Autodesk Inventor part; units mm, degrees
ref_plane "YZ Plane" through (0, 0, 0) normal (1, 0, 0) x (0, 1, 0)
ref_plane "XZ Plane" through (0, 0, 0) normal (0, 1, 0) x (-1, 0, 0)
ref_plane "XY Plane" through (0, 0, 0) normal (0, 0, 1) x (1, 0, 0)
sketch "Skizze1" plane through (0, 0, 0) normal (0, 0, 1) x (1, 0, 0)
  line L0 (5, 5) -> (5, 50)
  line L1 (5, 50) -> (0, 50)
  line L2 (0, 50) -> (0, 0)
  line L3 (5, 5) -> (50, 5)
  line L4 (50, 5) -> (50, 0)
  line L5 (-10, 0) -> (60, 0)
  line L6 (0, -10) -> (0, 60)
  line L7 (0, 0) -> (50, 0)
  dimension "d3" = 5
  dimension "d4" = 5
  dimension "d5" = 50
  dimension "d6" = 50
extrude "Extrusion1" add sketch "Skizze1" along normal blind 25
sketch "Skizze3" plane through (0, 0, 0) normal (0, -1, 0) x (1, 0, 0)
  line L0 (0, 0) -> (0, 25)
  line L1 (50, 0) -> (0, 0)
  line L2 (50, 0) -> (50, 25)
  line L3 (50, 25) -> (40, 25)
  line L4 (40, 25) -> (40, 0)
  line L5 (40, 0) -> (50, 0)
  line L6 (50, 0) -> (50, 25)
  dimension "d9" = 40
extrude "Extrusion2" cut sketch "Skizze3" against normal through all
sketch "Skizze4" plane through (0, 0, 0) normal (0, -1, 0) x (1, 0, 0)
  line L0 (40, 0) -> (40, 25)
  line L1 (40, 25) -> (0, 25)
  line L2 (0, 0) -> (0, 25)
  line L3 (5, 0) -> (5, 25)
  line L4 (40, 25) -> (5, 25)
  line L5 (5, 25) -> (5, 20.5)
  line L6 (5, 20.5) -> (40, 20.5)
  line L7 (40, 20.5) -> (40, 25)
  line L8 (5, 0) -> (40, 0)
  line L9 (40, 0) -> (40, 4.5)
  line L10 (40, 4.5) -> (5, 4.5)
  line L11 (5, 4.5) -> (5, 0)
  line L12 (0, 12.5) -> (40, 12.5)
  dimension "d12" = 16
extrude "Extrusion3" cut sketch "Skizze4" against normal through all contours L8 L3 L10 L0 | L6 L3 L1 L0
sketch "Skizze5" plane through (0, 0, 0) normal (0, -1, 0) x (1, 0, 0)
  line L0 (40, 4.5) -> (40, 20.5)
  line L1 (0, 0) -> (0, 25)
  line L2 (0, 12.5) -> (40, 12.5)
  point P0 (11, 12.5)
  point P1 (29, 12.5)
  dimension "d15" = 18
  dimension "d16" = 11
hole "Bohrung1" at (11, 0, 12.5) at (29, 0, 12.5) direction (0, 1, 0) diameter 4.5 end through all
fillet "Rundung1" radius 4 2 edges at (5, 2.5, 20.5) (5, 2.5, 4.5)
sketch "Skizze6" plane through (5, 0, 0) normal (1, 0, 0) x (0, 0, -1)
  line L0 (0, 50) -> (-25, 50)
  line L1 (-0.5, 5) -> (-24.5, 5)
  line L2 (-12.5, 50) -> (-12.5, 10.6492)
  point P0 (-12.5, 40)
  point P1 (-12.5, 22)
  dimension "d25" = 10
  dimension "d26" = 18
hole "Bohrung2" at (5, 40, 12.5) at (5, 22, 12.5) direction (-1, 0, 0) diameter 4.5 end through all countersink diameter 9.2 countersink angle 90
properties part number "13_0204_014"
Source: CAD feature listing. Evaluate the final solid. Frame: model axes, mm. A direction names the side the tool comes from. Give positions to 0.01 mm unless a question says otherwise; leave off trailing zeros. Write each loop counter-clockwise with the first axis right and the second up, starting at its lowest first coordinate (ties: lowest second). Pieces come first, ordered by that corner, then holes. Notation, with made-up numbers: M 87.5,71 L 120.5,71 A6 ccw 120.5,76 Z; hole C -29,-24 d8. An arc over 180 degrees is marked long. Return JSON: item names as keys, results as strings. Group by question number.
1) Pin query (flat end, axial travel): P1, Ø1.5, axis at y = 14, z = 22, coming from the -X side; P2, Ø5.5, axis at x = 25, y = 3.5, coming from the -Z side; P3, Ø5.5, axis at x = 28, y = 1.5, coming from the +Z side; P4, Ø4, axis at y = 40, z = 12.5, coming from the +X side. Return the tip coordinate at first contact, or that it passes through.
2) Cut plane A-A, the plane z = 12.5. Output: boundary loops of the cut face in (x, y), plus the area to 3 significant figures.
3) Pull-direction query (Y, two-part tool) for faces 5 (the face through (1.306, 24.196, 12.988)), 6 (the face through (3, 50, 12)), 7 (the face through (0, 25, 12)); classes: pulls with the +Y half, pulls with the -Y half, needs draft (parallel to the pull), parting line crosses it, or undercut.
4) Cut plane B-B, the plane y = 22. Output: boundary loops of the cut face in (x, z), plus the area to 3 significant figures.
5) Cut plane D-D, the plane z = 5.75. Output: boundary loops of the cut face in (x, y).
6) Set-up query: faces 1 (the face through (25, 2, 4.5)), 2 (the face through (22, 5, 12)), 3 (the face through (24, 2, 20.5)), 4 (the face through (40, 2, 13)). Return all of +Z, -Z, +X, -X, +Y, -Y with unobstructed straight access to the full face (end or side cutting, diameter ignored); none if empty.
7) Material intervals for line 1 along Y through (x, z) = (1.3, 12.5); line 2 along X through (y, z) = (1.2, 12.5); line 3 along Z through (x, y) = (11, 3), sorted ascending. Write a range as [from, to].
8) Cut plane C-C, the plane x = 29. Output: boundary loops of the cut face in (y, z).
Recorded:
{
 "1": {"P1": "stops at x = 0", "P2": "stops at z = 4.5", "P3": "stops at z = 20.5", "P4": "passes through"},
 "2": {"outline": "M 0,0 L 8.75,0 L 8.75,5 L 5,5 L 5,17.4 L 2.65,19.75 L 0,19.75 Z; M 0,24.25 L 2.65,24.25 L 5,26.6 L 5,35.4 L 2.65,37.75 L 0,37.75 Z; M 0,42.25 L 2.65,42.25 L 5,44.6 L 5,50 L 0,50 Z; M 13.25,0 L 26.75,0 L 26.75,5 L 13.25,5 Z; M 31.25,0 L 40,0 L 40,5 L 31.25,5 Z", "area": "324 mm²"},
 "3": {"face 5": "undercut", "face 6": "pulls with the +Y half", "face 7": "needs draft"},
 "4": {"outline": "M 0,0 L 5,0 L 5,7.9 L 2.65,10.25 L 0,10.25 Z; M 0,14.75 L 2.65,14.75 L 5,17.1 L 5,25 L 0,25 Z", "area": "97.0 mm²"},
 "5": {"outline": "M 0,0 L 40,0 L 40,5 L 5,5 L 5,50 L 0,50 Z"},
 "6": {"face 1": "-Z, +X, +Y, -Y", "face 2": "+Z, -Z, +X, +Y", "face 3": "+Z, +X, +Y, -Y", "face 4": "+Z, -Z, +X, +Y, -Y"},
 "7": {"line 1": "y = [0, 19.75], [24.25, 37.75], [42.25, 50]", "line 2": "x = [0, 8.75], [13.25, 26.75], [31.25, 40]", "line 3": "z = [4.5, 10.25], [14.75, 20.5]"},
 "8": {"outline": "M 0,4.5 L 5,4.5 L 5,10.25 L 0,10.25 Z; M 0,14.75 L 5,14.75 L 5,20.5 L 0,20.5 Z"}
}
